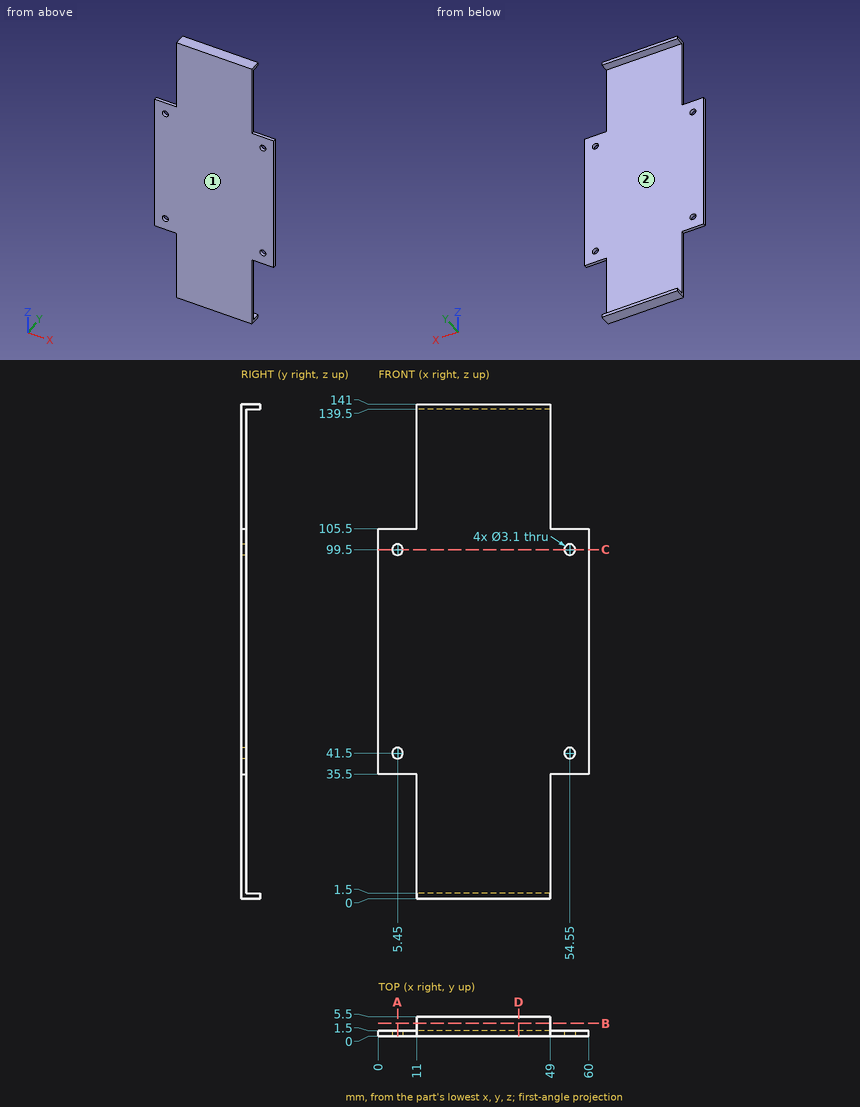
Geometry: see drawing. Coordinates: mm, zero at the bounding-box minimum. Coordinates: 2 decimals unless noted, no trailing zeros. Order: outer loops, then holes, each group sorted by start corner. A loop starts at its lowest first (then second) coordinate and runs counter-clockwise, first axis right, second up. Notation, with made-up numbers: M -27.5,68 L 6.5,68 A19 ccw 6.5,95 Z; hole C 16.5,12 d4. An arc over 180 degrees is marked long. Answer in a Markdown table with one row per item. Add a question column.
Q1. Contact query for flat-ended pins moving along their axis: P1, Ø3.5, axis at x = 5.45, z = 41.5, coming from the -Y side; P2, Ø2, axis at y = 3.5, z = 112.5, coming from the +X side; P3, Ø5, axis at x = 54.55, z = 41.5, coming from the +Y side; P4, Ø1.6, axis at y = 1.5, z = 25, coming from the +X side. Output: stop coordinate, or through.
Q2. Section query D-D on x = 40. Return the cut outline in (y, z).
Q3. Section query C-C on z = 99.5. Return the cut outline in (x, y).
Q4. Mould query, pull axis Z, two halves, no side actions, for the marked faces 1 and 2. Classes: released by +Z, released by -Z, zero draft, split by the parting line, or undercut.
Q5. Section query A-A on x = 5.45. Return the cut outline in (y, z), and give its area (3 significant figures).
Q6. Line query: L1, parallel to Z at x = 54.55, y = 0.75; L2, parallel to X at y = 1.1, z = 41.5; L3, parallel to Z at x = 32.5, y = 3.95. Output: solid intervals per line, ascending.
Q7. Section query B-B on y = 3.6. Return the cut outline in (x, z).
Completed:
| question | item | result |
|---|---|---|
| 1 | P1 | stops at y = 0 |
| 1 | P2 | passes through |
| 1 | P3 | stops at y = 1.5 |
| 1 | P4 | stops at x = 49 |
| 2 | outline | M 0,0 L 5.5,0 L 5.5,1.5 L 1.5,1.5 L 1.5,139.5 L 5.5,139.5 L 5.5,141 L 0,141 Z |
| 3 | outline | M 0,0 L 3.9,0 L 3.9,1.5 L 0,1.5 Z; M 7,0 L 53,0 L 53,1.5 L 7,1.5 Z; M 56.1,0 L 60,0 L 60,1.5 L 56.1,1.5 Z |
| 4 | face 1 | zero draft |
| 4 | face 2 | undercut |
| 5 | outline | M 0,35.5 L 1.5,35.5 L 1.5,39.95 L 0,39.95 Z; M 0,43.05 L 1.5,43.05 L 1.5,97.95 L 0,97.95 Z; M 0,101.05 L 1.5,101.05 L 1.5,105.5 L 0,105.5 Z |
| 5 | area | 95.7 mm2 |
| 6 | L1 | z = 35.5 to 39.95, 43.05 to 97.95, 101.05 to 105.5 |
| 6 | L2 | x = 0 to 3.9, 7 to 53, 56.1 to 60 |
| 6 | L3 | z = 0 to 1.5, 139.5 to 141 |
| 7 | outline | M 11,0 L 49,0 L 49,1.5 L 11,1.5 Z; M 11,139.5 L 49,139.5 L 49,141 L 11,141 Z |
